Work out the finished part from the listing and answer in its coordinate system (mm). Face numbers are marked on the shaded views. Give positions to 0.01 mm unless a question says otherwise; leave off trailing zeros. Loops run counter-clockwise (first coordinate to the right, second up) from the corner with the lowest first, then second, coordinate; pieces in that order, holes last. Notation, with made-up numbers: (-28, 5) - (24, 5) arc R19 cw to (24, 41) - close; hole circle Ø6 at (83.25, -13). An arc over 180 degrees is marked (long way). Use CSV: the item, a comma, the result in double quotes.
from build123d import *

# Parameters (mm, degrees)
SKETCH1_W           = 342.9
SKETCH1_H           = 127
BOSS_EXTRUDE1_DEPTH = 12.7
DRAFT1_ANGLE        = -45
CUT_EXTRUDE1_DEPTH  = 5.08
SKETCH3_W           = 23.368
SKETCH3_H           = 127
CUT_EXTRUDE2_DEPTH  = 5.08
SKETCH4_W           = 172.212
SKETCH4_H           = 26.162
CUT_EXTRUDE3_DEPTH  = 5.08


with BuildPart() as part:
    # Sketch1 → Boss-Extrude1 (new body)
    with BuildSketch(Plane(origin=(0, 0, 0), x_dir=(1, 0, 0), z_dir=(0, 1, 0))):
        Rectangle(SKETCH1_W, SKETCH1_H)
    extrude(amount=BOSS_EXTRUDE1_DEPTH)

    # Draft1
    draft1_faces = [part.faces().sort_by_distance(p)[0] for p in [
        (0, 6.35, -63.5),
        (-171.45, 6.35, 0),
        (171.45, 6.35, 0),
        (0, 6.35, 63.5),
    ]]
    draft(draft1_faces, Plane(origin=(0, 0, 0), x_dir=(0, 0, -1), z_dir=(0, -1, 0)), DRAFT1_ANGLE)

    # Sketch2 → Cut-Extrude1 (cut)
    with BuildSketch(Plane(origin=(0, 12.7, 0), x_dir=(1, 0, 0), z_dir=(0, 1, 0))):
        with BuildLine():
            Line((-19.431, -63.5), (19.431, -63.5))
            Line((19.431, -63.5), (19.431, -30.988))
            ThreePointArc((19.431, -30.988), (12.827, -24.384), (6.223, -30.988))
            Line((6.223, -30.988), (-6.223, -30.988))
            ThreePointArc((-6.223, -30.988), (-12.827, -24.384), (-19.431, -30.988))
            Line((-19.431, -30.988), (-19.431, -63.5))
        make_face()
    extrude(amount=-CUT_EXTRUDE1_DEPTH, mode=Mode.SUBTRACT)

    # Sketch3 → Cut-Extrude2 (cut)
    with BuildSketch(Plane(origin=(0, 12.7, 0), x_dir=(1, 0, 0), z_dir=(0, 1, 0))):
        with Locations((-12.446, 0)):
            Rectangle(SKETCH3_W, SKETCH3_H)
    extrude(amount=-CUT_EXTRUDE2_DEPTH, mode=Mode.SUBTRACT)

    # Sketch4 → Cut-Extrude3 (cut)
    with BuildSketch(Plane(origin=(0, 12.7, 0), x_dir=(1, 0, 0), z_dir=(0, 1, 0))):
        with Locations((85.344, 50.419)):
            Rectangle(SKETCH4_W, SKETCH4_H)
    extrude(amount=-CUT_EXTRUDE3_DEPTH, mode=Mode.SUBTRACT)


solid = part.part
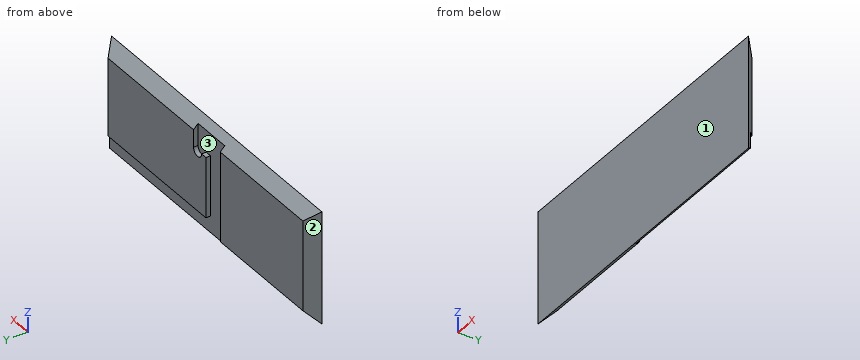
Item 1: Find the intervals of material crossed by line 1 (X direction, y = 10, z = -6); line 2 (Y direction, x = -20.5, z = 35.5); line 3 (X direction, y = 12, z = -1), in increasing order.
Determined:
line 1,"x = -161.45 to -24.13, -0.76 to 161.45"
line 2,"y = 0 to 7.62"
line 3,"x = -159.45 to -24.13, -0.76 to 159.45"
Item 2: A cutting plane is placed at C-C on x = -149. Determine the outline of the cut face in (y, z), and give its area (3 significant figures).
Determined:
outline,"(0, -63.5) - (12.7, -50.8) - (12.7, 50.8) - (0, 63.5) - close"
area,"1,450 mm²"
Item 3: Given P1, Ø1.5, axis at y = 9.5, z = 46.5, coming from the -X side; P2, Ø3, axis at x = 83, y = 6, coming from the -Z side; P3, Ø5, axis at y = 10, z = -35.5, coming from the -X side, each flat-ended and moving along its own axis, determine where each tip first touches the part or whether it passes through.
Determined:
P1,"stops at x = -162.7"
P2,"stops at z = -59"
P3,"stops at x = -163.95"
Item 4: The mould has two halves that part along X. Classify the marked faces 1, 2 and 3: pulls with the +X half, pulls with the -X half, needs draft (parallel to the pull), parting line crosses it, or undercut.
Determined:
face 1,"needs draft"
face 2,"pulls with the -X half"
face 3,"undercut"
Item 5: A cutting plane is placed at B-B on z = -22.5. Determine the outline of the cut face in (x, y).
Determined:
outline,"(-171.45, 0) - (171.45, 0) - (158.75, 12.7) - (-0.76, 12.7) - (-0.76, 7.62) - (-24.13, 7.62) - (-24.13, 12.7) - (-158.75, 12.7) - close"
Item 6: A cutting plane is placed at D-D on x = 78. Determine the outline of the cut face in (y, z).
Determined:
outline,"(0, -63.5) - (7.62, -55.88) - (7.62, -37.34) - (12.7, -37.34) - (12.7, 50.8) - (0, 63.5) - close"
Item 7: A cutting plane is placed at A-A on y = 10.25. Determine the outline of the cut face in (x, z).
Determined:
outline,"(-161.2, -53.25) - (-24.13, -53.25) - (-24.13, 53.25) - (-161.2, 53.25) - close; (-0.76, -37.34) - (161.2, -37.34) - (161.2, 53.25) - (19.43, 53.25) - (19.43, 30.99) arc R6.6 cw to (6.22, 30.99) - (-0.76, 30.99) - close"
